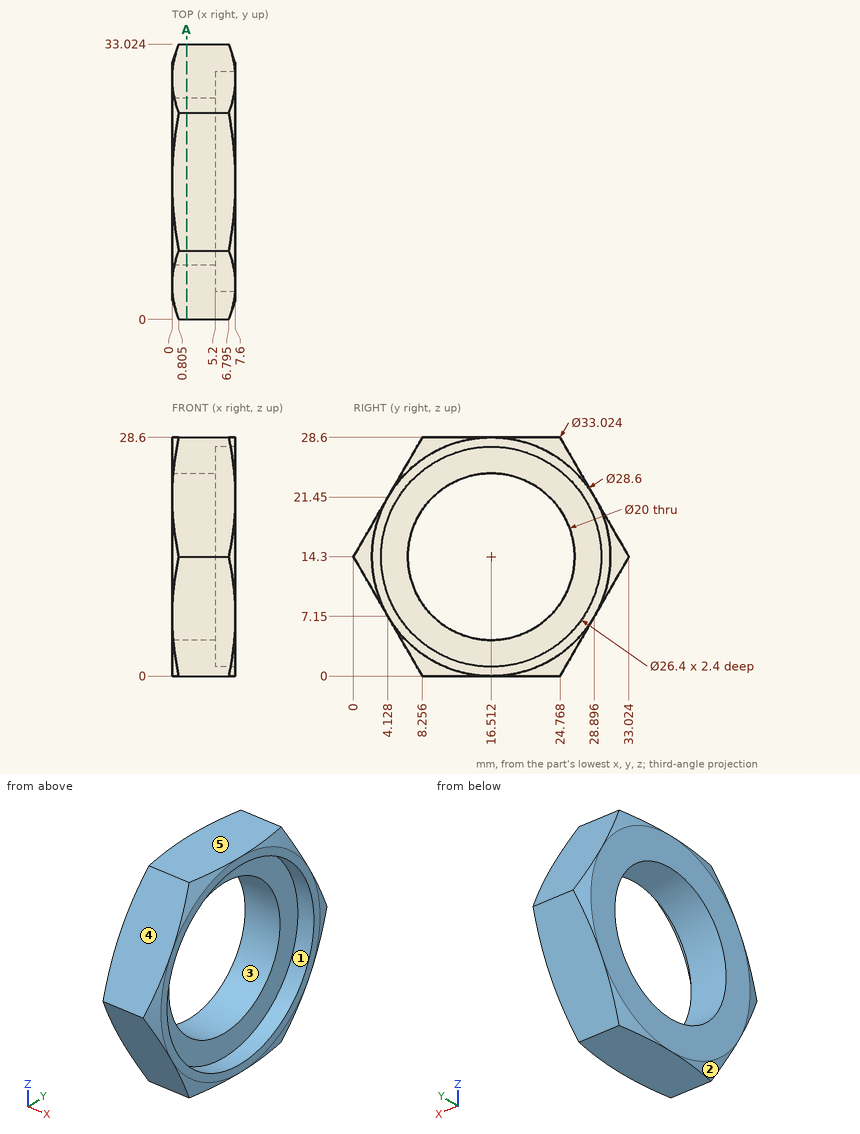
Check sheet for the drawn part. Datum: minimum x, y, z corner. Units: mm. A direction names the side the tool comes from. Round coordinates to 2 decimals unless told otherwise and drop trailing zeros. Write each loop counter-clockwise with the first axis right and the second up, starting at its lowest first coordinate (ties: lowest second). Pieces come first, ordered by that corner, then holes. Notation, with made-up numbers: (-22, 67) -> (-15, 67) arc R17 cw to (-15, 76) -> close; hole circle Ø5 at (3, -0.5). An arc over 180 degrees is marked (long way). Put each result on its own line as item: value.
(1) Tool access check on the marked faces 1 and 2. Record the directions out of +Z, -Z, +X, -X, +Y, -Y that give a thin tool (end or side, any length) a straight path to the whole face; none if there is none.
Values found:
face 1: +X
face 2: -Z, -X, -Y
(2) Mould release check, pull along Y, two halves, no side actions. Record for the marked faces 3, 4 and 5: released by +Y, released by -Y, zero draft, split by the parting line, or undercut.
Values found:
face 3: undercut
face 4: released by -Y
face 5: zero draft
(3) Go/stop test with flat-tipped pins: pin 1 Ø1.5 at (x, z) = (5.5, 22.5) entering from -Y; pin 2 Ø12 at (y, z) = (4, 7) entering from -X; pin 3 Ø4 at (y, z) = (8, 16.5) entering from +X. Record where each tip stops, or that it passes through.
Values found:
pin 1: stops at y = 4.3
pin 2: stops at x = 0
pin 3: stops at x = 5.2
(4) Material ranges on line 1 (X direction, y = 27.5, z = 16.5); line 2 (Z direction, x = 5.75, y = 25) (1 decimal); line 3 (Z direction, x = 2.75, y = 21) (1 decimal), recorded low to high.
Values found:
line 1: x = 0 to 5.2
line 2: z = 0.4 to 4.2, 24.4 to 28.2
line 3: z = 0 to 5.4, 23.2 to 28.6
(5) Sectioned sample at A-A (x = 1.75). Enter the section's corners in (y, z) (1 decimal).
Values found:
outline: (0, 14.3) -> (8.3, 0) -> (24.8, 0) -> (33, 14.3) -> (24.8, 28.6) -> (8.3, 28.6) -> close; hole circle Ø20 at (16.5, 14.3)
